Could you check a few things on this model? Use its own coordinates, in mm. Coordinates: 2 decimals unless noted, no trailing zeros. Order: outer loops, then holes, each group sorted by start corner. A loop starts at its lowest first (then second) coordinate and runs counter-clockwise, first axis right, second up. Notation, with made-up numbers: (45, 19) - (50, 19) arc R15 ccw to (50, 41) - close; hole circle Ø2 at (44, 77). An arc over 180 degrees is marked (long way). Answer as CSV lines item,"result". Start each with the question number.
1. I want a section at B-B, the plane x = -43. List the corners of the cut face in (y, z) for me, and give its area (3 significant figures).
2. Thinking about a two-plate mould opening in Z: for faces 1 (the face through (48.37, 3.7, -46.55)), 2 (the face through (66.922, 3.698, -51.135)), 3 (the face through (1, 4, -61.059)), 4 (the face through (-53.172, 3.698, -44.805)), which applies, released by +Z, released by -Z, zero draft, split by the parting line, or undercut?
3. I want a section at D-D, the plane z = -9. List the corners of the cut face in (x, y) for me, and give its area (3 significant figures).
4. I need wall thicknesses on probe 1 along Z at (x, y) = (-52, 3.5); probe 2 along X at (y, z) = (1.75, 48.5); probe 3 along Z at (x, y) = (51.5, 4.75). Which ranges of each line are inside material? Lowest first, please.
5. I want a section at C-C, the plane x = 2. List the corners of the cut face in (y, z) for me, and give its area (3 significant figures).
6. For pin 1 (1 mm diameter, centred on y = 4.5, z = 13.5, fed in from +X); pin 2 (4 mm diameter, centred on y = 4, z = -35.5, fed in from -X); pin 3 (13.5 mm diameter, centred on x = -48, z = -38.06, fed in from +Y), each with a flat end and sliding along its axis, tell me the tip position at first contact or that it passes through.
7. I want a section at A-A, the plane y = 3.25. List the corners of the cut face in (x, z) for me.
from build123d import *

# Parameters (mm, degrees)
SKETCH2_R           = 8.5
BOSS_EXTRUDE1_DEPTH = 7.5


with BuildPart() as part:
    # Sketch2 → Boss-Extrude1 (new body)
    # profile 1 of 2: a face of its own
    with BuildSketch(Plane(origin=(0, 0, 0), x_dir=(1, 0, 0), z_dir=(0, 1, 0))):
        with BuildLine():
            Line((0, 61.059418618), (-48, 61.059418618))
            ThreePointArc((-48, 61.059418618), (-66.745837136, 51.385843122), (-69.723042032, 30.502339493))
            Line((-69.723042032, 30.502339493), (-20.24936145, -61.347614016))
            ThreePointArc((-20.24936145, -61.347614016), (-11.792757299, -70.18724883), (0, -73.440581382))
            Line((0, -73.440581382), (0, -60.040453624))
            ThreePointArc((0, -60.040453624), (-8.5, -51.540453624), (0, -43.040453624))
            Line((0, -43.040453624), (0, 61.059418618))
        make_face()
        with Locations(Location((-48, 38.059418618, 0), (0, 0, 270))):
            Circle(SKETCH2_R, mode=Mode.SUBTRACT)
    # profile 2 of 2: a face of its own
    with BuildSketch(Plane(origin=(0, 0, 0), x_dir=(1, 0, 0), z_dir=(0, 1, 0))):
        with BuildLine():
            Line((48, 61.059418618), (0, 61.059418618))
            Line((0, 61.059418618), (0, -43.040453624))
            ThreePointArc((0, -43.040453624), (6.01040764, -45.530045984), (8.5, -51.540453624))
            ThreePointArc((8.5, -51.540453624), (6.01040764, -57.550861264), (0, -60.040453624))
            Line((0, -60.040453624), (0, -73.440581382))
            ThreePointArc((0, -73.440581382), (11.792757299, -70.18724883), (20.24936145, -61.347614016))
            Line((20.24936145, -61.347614016), (69.723042032, 30.502339493))
            ThreePointArc((69.723042032, 30.502339493), (66.745837136, 51.385843122), (48, 61.059418618))
        make_face()
        with Locations(Location((48, 38.059418618, 0), (0, 0, 270))):
            Circle(SKETCH2_R, mode=Mode.SUBTRACT)
    extrude(amount=BOSS_EXTRUDE1_DEPTH)


solid = part.part
Solved:
1,outline,"(0, -61.06) - (7.5, -61.06) - (7.5, -44.93) - (0, -44.93) - close; (0, -31.19) - (7.5, -31.19) - (7.5, 19.11) - (0, 19.11) - close"
1,area,"498 mm2"
2,face 1,"undercut"
2,face 2,"split by the parting line"
2,face 3,"released by -Z"
2,face 4,"undercut"
3,outline,"(-58.14, 0) - (58.14, 0) - (58.14, 7.5) - (-58.14, 7.5) - close"
3,area,"872 mm2"
4,probe 1,"z = -60.71 to -45.56, -30.56 to 2.4"
4,probe 2,"x = -27.17 to -7.94, 7.94 to 27.17"
4,probe 3,"z = -60.79 to -45.81, -30.31 to 3.33"
5,outline,"(0, -61.06) - (7.5, -61.06) - (7.5, 43.28) - (0, 43.28) - close; (0, 59.8) - (7.5, 59.8) - (7.5, 73.35) - (0, 73.35) - close"
5,area,"884 mm2"
6,pin 1,"stops at x = 46.29"
6,pin 2,"stops at x = -70.99"
6,pin 3,"passes through"
7,outline,"(-69.72, -30.5) arc R23 ccw to (-48, -61.06) - (48, -61.06) arc R23 ccw to (69.72, -30.5) - (20.25, 61.35) arc R23 ccw to (-20.25, 61.35) - close; hole circle Ø17 at (-48, -38.06); hole circle Ø17 at (0, 51.54); hole circle Ø17 at (48, -38.06)"
